Geometry check sheet. Reference: the model listing, model coordinates, mm. Face numbers are marked on the shaded views. Give positions to 0.01 mm unless a question says otherwise; leave off trailing zeros. Loops run counter-clockwise (first coordinate to the right, second up) from the corner with the lowest first, then second, coordinate; pieces in that order, holes last. Notation, with made-up numbers: (-9.5, 71.25) - (-2.5, 71.25) arc R18 ccw to (-2.5, 98.25) - close; hole circle Ø10 at (-21, -39). An arc over 180 degrees is marked (long way). Write item = value, one per line. Start each with the question number.
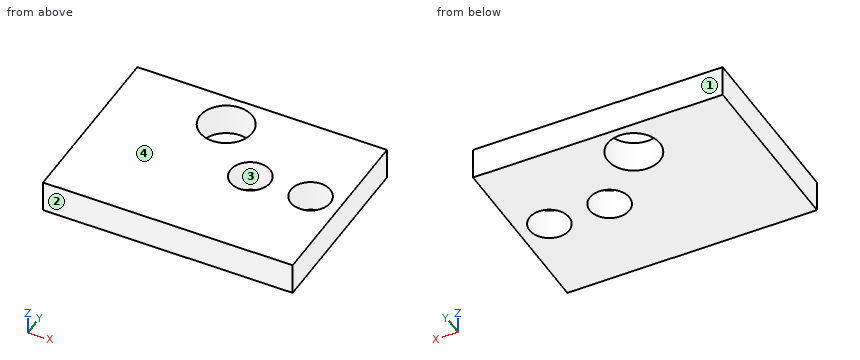
Autodesk Inventor part; units mm, degrees
ref_plane "YZ Plane" through (0, 0, 0) normal (1, 0, 0) x (0, 1, 0)
ref_plane "XZ Plane" through (0, 0, 0) normal (0, 1, 0) x (-1, 0, 0)
ref_plane "XY Plane" through (0, 0, 0) normal (0, 0, 1) x (1, 0, 0)
sketch "Sketch1" plane through (0, 0, 0) normal (0, 0, 1) x (1, 0, 0)
  point P0 (0, 0)
sketch "Sketch2" plane through (0, 0, 0) normal (0, 0, 1) x (1, 0, 0)
  line L0 (0, 0) -> (15.75, 0)
  line L1 (15.75, 0) -> (15.75, 11.43)
  line L2 (15.75, 11.43) -> (0, 11.43)
  line L3 (0, 11.43) -> (0, 0)
  dimension "d0" = 15.75
  dimension "d1" = 11.43
extrude "Extrusion1" add sketch "Sketch2" along normal blind 2
sketch "Sketch3" plane through (0, 0, 2) normal (0, 0, 1) x (1, 0, 0)
  line L0 (15.75, 11.43) -> (0, 11.43)
  line L1 (0, 11.43) -> (6.73, 11.43)
  line L2 (0, 11.43) -> (6.73, 11.43) construction
  line L3 (6.73, 11.43) -> (6.73, 9.27)
  circle A0 centre (6.73, 9.27) radius 1.651
  line L4 (15.75, 11.43) -> (13.84, 11.43)
  line L5 (15.75, 11.43) -> (17.66, 11.43) construction
  line L6 (13.84, 11.43) -> (13.84, 5.84)
  line L7 (13.84, 5.84) -> (10.04, 5.84)
  circle A1 centre (10.04, 5.84) radius 1.25
  circle A2 centre (13.84, 5.84) radius 1.25
  point P0 (0, 0)
  dimension "d4" = 6.73
  dimension "d5" = 0
  dimension "d6" = 2.16
  dimension "d7" = 90
  dimension "d8" = 3.302
  dimension "d9" = 1.91
  dimension "d10" = 180
  dimension "d11" = 5.59
  dimension "d12" = 90
  dimension "d13" = 3.8
  dimension "d14" = 90
  dimension "d15" = 2.5
  dimension "d16" = 2.5
extrude "Extrusion2" cut sketch "Sketch3" against normal blind 2
properties part number "SensorPCB"
1) Cross-section at A-A on x = 13.84. Enter the section's corners in (y, z), and give its area (3 significant figures).
2) Cross-section at C-C on y = 9.27. Enter the section's corners in (x, z).
3) Material ranges on line 1 along X through (y, z) = (9.27, 0.4); line 2 along Y through (x, z) = (6.73, 1.6); line 3 along Y through (x, z) = (13.84, 1.5), recorded low to high.
4) Cross-section at D-D on z = 0.9. Enter the section's corners in (x, y).
5) Release check for a two-part mould opening along Y. For the marked faces 1, 2, 3 and 4 record: pulls with the +Y half, pulls with the -Y half, needs draft (parallel to the pull), parting line crosses it, or undercut.
6) Cross-section at B-B on y = 5.84. Enter the section's corners in (x, z), and give its area (3 significant figures).
7) Gauge pin test, flat ends, axial feed: P1, Ø1, axis at x = 4.5, z = 0.5, coming from the -Y side; P2, Ø2.5, axis at x = 6.73, y = 9.27, coming from the -Z side. Record the tip position at first contact, or that the pin passes through.
Checked values:
q1.outline = (0, 0) - (4.59, 0) - (4.59, 2) - (0, 2) - close; (7.09, 0) - (11.43, 0) - (11.43, 2) - (7.09, 2) - close
q1.area = 17.9 mm²
q2.outline = (0, 0) - (5.08, 0) - (5.08, 2) - (0, 2) - close; (8.38, 0) - (15.75, 0) - (15.75, 2) - (8.38, 2) - close
q3.line_1 = 0 to 5.08, 8.38 to 15.75
q3.line_2 = 0 to 7.62, 10.92 to 11.43
q3.line_3 = 0 to 4.59, 7.09 to 11.43
q4.outline = (0, 0) - (15.75, 0) - (15.75, 11.43) - (0, 11.43) - close; hole circle Ø3.3 at (6.73, 9.27); hole circle Ø2.5 at (10.04, 5.84); hole circle Ø2.5 at (13.84, 5.84)
q5.face_1 = pulls with the +Y half
q5.face_2 = pulls with the -Y half
q5.face_3 = undercut
q5.face_4 = needs draft
q6.outline = (0, 0) - (8.79, 0) - (8.79, 2) - (0, 2) - close; (11.29, 0) - (12.59, 0) - (12.59, 2) - (11.29, 2) - close; (15.09, 0) - (15.75, 0) - (15.75, 2) - (15.09, 2) - close
q6.area = 21.5 mm²
q7.P1 = 0
q7.P2 = through
